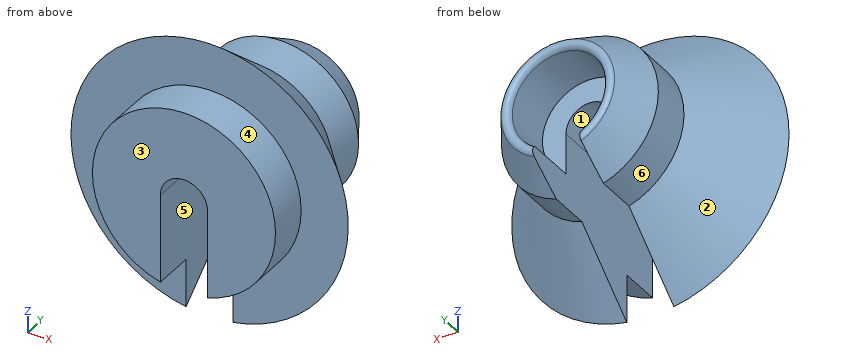
from build123d import *

# Parameters (mm, degrees)
FILLET1_R          = 0.5
SKETCH3_W          = 4.5
SKETCH3_H          = 28.736220623
CUT_EXTRUDE1_DEPTH = 28


with BuildPart() as part:
    # Sketch2 → Revolve1 (revolve)
    with BuildSketch(Plane.XY, mode=Mode.PRIVATE) as revolve1_sk:
        Polygon((-2.25, 13.5), (-2.25, 0), (-8.75, 0), (-8.75, 4), (-13.25, 4), (-7.5, 11), (-7.5, 15), (-4.5, 20), (-4.5, 13.5), align=None)
    revolve(revolve1_sk.sketch.rotate(Axis((0, 0, 0), (0, 1, 0)), 270), axis=Axis((0, 0, 0), (0, 1, 0)))

    # Fillet1
    fillet1_edges = [part.edges().sort_by_distance(p)[0] for p in [
        (0, 20, 4.5),
    ]]
    fillet(fillet1_edges, radius=FILLET1_R)

    # Sketch3 → Cut-Extrude1 (cut)
    with BuildSketch(Plane.XZ):
        with Locations((0, -14.368110312)):
            Rectangle(SKETCH3_W, SKETCH3_H)
    extrude(amount=-CUT_EXTRUDE1_DEPTH, mode=Mode.SUBTRACT)


solid = part.part
The model under review builds one solid part; all positions refer to its coordinate system, in mm. Face numbers are marked on the shaded views. A direction names the side the tool comes from. Round coordinates to 2 decimals unless told otherwise and drop trailing zeros. Loops run counter-clockwise (first coordinate to the right, second up) from the corner with the lowest first, then second, coordinate; pieces in that order, holes last. Notation, with made-up numbers: (3.25, 14.5) - (62.25, 14.5) arc R11 cw to (62.25, 19.5) - close; hole circle Ø7 at (69, 44.5). An arc over 180 degrees is marked (long way). Use CSV: the item, a comma, the result in double quotes.
(1) Take a section at A-A, the plane y = 2. Give the boundary of the cut face in (x, z), plus the area to 3 significant figures.
Working result:
outline,"(-2.25, -8.46) - (-2.25, 0) arc R2.25 cw to (2.25, 0) - (2.25, -8.46) arc R8.75 ccw (long way) to start"
area,"194 mm^2"
(2) For line 1 (X direction, y = 14.5, z = 0); line 2 (X direction, y = 8, z = -9); line 3 (Z direction, x = 0, y = 14.5), list the stretches that pass through material, from the lowest coordinate up.
Working result:
line 1,"x = -7.5 to -4.5, 4.5 to 7.5"
line 2,"x = -4.28 to -2.25, 2.25 to 4.28"
line 3,"z = 4.5 to 7.5"
(3) Machinability: for the marked faces 4, 5 and 6, which of the approach directions +Z, -Z, +X, -X, +Y, -Y give a long, thin tool a straight path to every point of the face, cutting with its end or side? Answer none if there is none.
Working result:
face 4,"-Y"
face 5,"-Z, +Y, -Y"
face 6,"+Y"
(4) Take a section at B-B, the plane y = 5. Give the boundary of the cut face in (x, z).
Working result:
outline,"(-2.25, -12.22) - (-2.25, 0) arc R2.25 cw to (2.25, 0) - (2.25, -12.22) arc R12.43 ccw (long way) to start"
(5) The part is to be moulded in two halves that separate along X. For the marked faces 1, 2 and 3, say which applies: pulls with the +X half, pulls with the -X half, needs draft (parallel to the pull), parting line crosses it, or undercut.
Working result:
face 1,"undercut"
face 2,"parting line crosses it"
face 3,"needs draft"
(6) Clearance check with flat-ended pins moving along their axes: P1, Ø6, axis at x = 1, y = 9.5, coming from the +Z side; P2, Ø10.5, axis at y = 13.5, z = -8, coming from the +X side; P3, Ø5, axis at x = -9.5, y = 8.5, coming from the +Z side; P4, Ø2, axis at x = -9, y = 12, coming from the +Z side. State where each tip first meets the part, or that it passes through.
Working result:
P1,"stops at z = 11.16"
P2,"stops at x = 7.47"
P3,"stops at z = 7.84"
P4,"passes through"
